```python
from build123d import *

# Parameters (mm, degrees)
F0_R        = 1.5
F1_DEPTH    = 22
F2_T1_DEPTH = 165.7438624109
F3_DEPTH    = 10


# Not quite as in the source:
# - a fillet or chamfer that OpenCascade refuses, or shapes differently, is made with other operations: its cross-section is extruded or revolved along the edge and cut away or added


with BuildPart() as f1:
    # F0 (on Top) → F1 (new body)
    with BuildSketch(Plane.XY):
        with BuildLine():
            ThreePointArc((-76.7321565298, 10.8823781538), (-76.533256864, 12.202892845), (-76.3116336523, 13.5197843663))
            Line((-76.3116336523, 13.5197843663), (-84.2766601783, 11.9523616575))
            Line((-84.2766601783, 11.9523616575), (-76.7321565298, 10.8823781538))
        make_face()
        with BuildLine():
            ThreePointArc((-76.3116336523, 13.5197843663), (-71.9683443093, 28.7542591172), (-64.6180706596, 42.7873222372))
            Line((-64.6180706596, 42.7873222372), (-72.9558862286, 48.3082670421))
            ThreePointArc((-72.9558862286, 48.3082670421), (-81.8018975861, 31.0596128649), (-86.633079953, 12.2865559801))
            Line((-86.633079953, 12.2865559801), (-84.2766601783, 11.9523616575))
            Line((-84.2766601783, 11.9523616575), (-76.3116336523, 13.5197843663))
        make_face()
        with Locations((-79.5430595227, 21.8895336125)):
            Circle(F0_R, mode=Mode.SUBTRACT)
        with Locations((-72.3838330612, 39.5832124944)):
            Circle(F0_R, mode=Mode.SUBTRACT)
        with BuildLine():
            ThreePointArc((-64.6180706596, 42.7873222372), (-64.076826103, 43.5936962939), (-63.5255193134, 44.3932246628))
            Line((-63.5255193134, 44.3932246628), (-71.7223605151, 50.1213826839))
            ThreePointArc((-71.7223605151, 50.1213826839), (-72.3448036647, 49.218689364), (-72.9558862286, 48.3082670421))
            Line((-72.9558862286, 48.3082670421), (-64.6180706596, 42.7873222372))
        make_face()
        with BuildLine():
            ThreePointArc((-76.8036989266, 10.365415148), (-76.7683628871, 10.6239568725), (-76.7321565298, 10.8823781538))
            Line((-76.7321565298, 10.8823781538), (-84.2766601783, 11.9523616575))
            Line((-84.2766601783, 11.9523616575), (-86.7454235032, 11.466538329))
            ThreePointArc((-86.7454235032, 11.466538329), (-86.9376476661, 9.9043131153), (-87.1017395415, 8.3388829496))
            Line((-87.1017395415, 8.3388829496), (-76.8036989266, 10.365415148))
        make_face()
        with BuildLine():
            Line((-86.7454235032, 11.466538329), (-84.2766601783, 11.9523616575))
            Line((-84.2766601783, 11.9523616575), (-86.633079953, 12.2865559801))
            ThreePointArc((-86.633079953, 12.2865559801), (-86.6902213195, 11.8766799899), (-86.7454235032, 11.466538329))
        make_face()
        with Locations((-72.3838330612, 39.5832124944)):
            Circle(F0_R)
        with Locations((-79.5430595227, 21.8895336125)):
            Circle(F0_R)
    extrude(amount=F1_DEPTH)

    # F2: chamfer of 17 x 30 on 1 edges, made by hand

    # F2_s2 → F2_t1 (cut)
    with BuildSketch(Plane(origin=(-158.4380449398, -31.1787272483, 0), x_dir=(0, 0, 1), z_dir=(0.9811820369, 0.1930849823, 0))):
        Polygon((5, -25), (22, -55), (22, -25), align=None)
    extrude(amount=F2_T1_DEPTH, mode=Mode.SUBTRACT)

    # F0 (on Top) → F3 (cut)
    with BuildSketch(Plane.XY):
        with Locations((-72.3838330612, 39.5832124944)):
            Circle(F0_R)
        with Locations((-79.5430595227, 21.8895336125)):
            Circle(F0_R)
    extrude(amount=F3_DEPTH, mode=Mode.SUBTRACT)


solid = f1.part
```
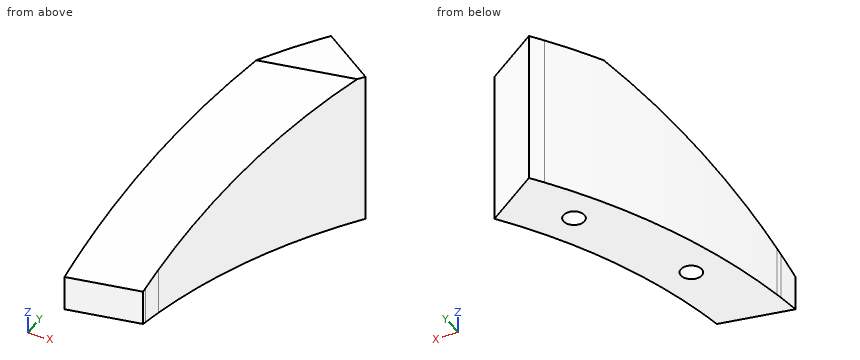
Check sheet for the modelled part. Datum: model origin and axes. Units: mm. Coordinates: 2 decimals unless noted, no trailing zeros. Order: outer loops, then holes, each group sorted by start corner. A loop starts at its lowest first (then second) coordinate and runs counter-clockwise, first axis right, second up. Notation, with made-up numbers: M -0.75,-6 L 12.25,-6 A27 cw 12.25,11 Z; hole C 66,-40 d9. An arc over 180 degrees is marked long. Write each question's results on one line, items separated by ' | '. Start each with the question number.
1. Cross-section at A-A on z = 9. Record the cut outline in (x, y), and give its area (3 significant figures).
2. Cross-section at D-D on y = 34. Record the cut outline in (x, z).
3. Cross-section at B-B on x = -74.5. Record the cut outline in (y, z).
4. Cross-section at C-C on z = 14.5. Record the cut outline in (x, y), and give its area (3 significant figures).
5. Material ranges on probe 1 along X at (y, z) = (22, 9.25); probe 2 along Y at (x, z) = (-69.5, 13); probe 3 along Y at (x, z) = (-78.5, 10.5), recorded low to high.
6. Go/stop test with flat-tipped pins: P1, Ø3, axis at x = -84.5, z = 12.5, coming from the -Y side; P2, Ø1.5, axis at x = -72, y = 40, coming from the -Z side; P3, Ø8, axis at y = 35, z = 7.5, coming from the -X side. Record where each tip stops, or that it passes through.
Checks:
1) outline: M -86.07,15.74 L -75.42,17.83 A77.5 cw -63.53,44.39 L -71.72,50.12 A87.5 ccw Z; hole C -79.54,21.89 d3; hole C -72.38,39.58 d3 | area: 320 mm²
2) outline: M -80.62,0 L -69.64,0 L -69.64,17.36 L -80.62,18.56 Z
3) outline: M 21.35,0 L 45.89,0 L 45.89,22 L 41.39,22 L 21.35,10.86 Z
4) outline: M -83.51,26.13 L -72.12,28.37 A77.5 cw -63.53,44.39 L -71.72,50.12 A87.5 ccw Z | area: 225 mm²
5) probe 1: x = -84.69 to -81.04, -78.05 to -74.31 | probe 2: y = 34.29 to 48.57 | probe 3: y = 19.92 to 38.65
6) P1: stops at y = 19.63 | P2: stops at z = 10 | P3: stops at x = -81.82
